from build123d import *

# Parameters (mm, degrees)
SKETCH_R        = 2
SKETCH_W        = 22
SKETCH_H        = 48
PAD_DEPTH       = 7
SKETCH001_W     = 29.4
SKETCH001_H     = 53.5
POCKET_DEPTH    = 6
SKETCH002_R     = 3.5
POCKET001_DEPTH = 3


with BuildPart() as part:
    # Sketch → Pad (new body)
    with BuildSketch(Plane.XY):
        with BuildLine():
            Line((3.870596, 38.332537), (15.423539, 30.665756))
            ThreePointArc((19, 24), (18.049408, 27.782307), (15.423539, 30.665756))
            Line((19, 24), (19, -24))
            ThreePointArc((15.423539, -30.665756), (18.049408, -27.782307), (19, -24))
            Line((15.423539, -30.665756), (3.870596, -38.332537))
            ThreePointArc((-3.870596, -38.332537), (0, -39.5), (3.870596, -38.332537))
            Line((-3.870596, -38.332537), (-15.423539, -30.665756))
            ThreePointArc((-19, -24), (-18.049408, -27.782307), (-15.423539, -30.665756))
            Line((-19, -24), (-19, 24))
            ThreePointArc((-15.423539, 30.665756), (-18.049408, 27.782307), (-19, 24))
            Line((-15.423539, 30.665756), (-3.870596, 38.332537))
            ThreePointArc((3.870596, 38.332537), (0, 39.5), (-3.870596, 38.332537))
        make_face()
        with Locations((0, 32.5)):
            Circle(SKETCH_R, mode=Mode.SUBTRACT)
        with Locations((0, -32.5)):
            Circle(SKETCH_R, mode=Mode.SUBTRACT)
        Rectangle(SKETCH_W, SKETCH_H, mode=Mode.SUBTRACT)
    extrude(amount=PAD_DEPTH)

    # Sketch001 → Pocket (cut)
    with BuildSketch(Plane.XY):
        Rectangle(SKETCH001_W, SKETCH001_H)
    extrude(amount=POCKET_DEPTH, mode=Mode.SUBTRACT)

    # Sketch002 (on Face4 of Pocket) → Pocket001 (cut)
    with BuildSketch(Plane(origin=(0, 0, 0), x_dir=(1, 0, 0), z_dir=(0, 0, -1))):
        with Locations((0, -32.5)):
            Circle(SKETCH002_R)
        with Locations((0, 32.5)):
            Circle(SKETCH002_R)
    extrude(amount=-POCKET001_DEPTH, mode=Mode.SUBTRACT)


solid = part.part
Geometry: final body of the model. Coordinates: model frame, mm. A direction names the side the tool comes from. Give positions to 0.01 mm unless a question says otherwise; leave off trailing zeros. Loops run counter-clockwise (first coordinate to the right, second up) from the corner with the lowest first, then second, coordinate; pieces in that order, holes last. Notation, with made-up numbers: (53, -24) - (76, -24) arc R12 cw to (76, -3) - close; hole circle Ø9 at (81.25, 63). An arc over 180 degrees is marked (long way). One line per question, with ' | ' between items. Start each with the question number.
(1) Ray query, line 1 (X direction, y = 23.5, z = 5); line 2 (Y direction, x = 1.5, z = 5); line 3 (Z direction, x = -12, y = 17). Return the intervals inside material, ascending. Write a range as from..to.
(2) Section query B-B on y = 0.5. Return loops of the section in (x, z).
(3) Reachability of faces 5 (the flat face through (2, 34, 3)), 6 (the flat face through (9.57, 34.55, 3.45)) from +Z, -Z, +X, -X, +Y, -Y: full face, straight path, thin tool, end or side. Return the list, or none.
(4) Section query A-A on x = 0. Return loops of the section in (y, z).
(5) Pull-direction query (Y, two-part tool) for faces 1 (the flat face through (-9.728, 34.445, 3.451)), 2 (the cylindrical face through (0, 29, 1)), 3 (the flat face through (19, 0, 3)), 4 (the cylindrical face through (-0.1, -39.5, 3.5)); classes: released by +Y, released by -Y, zero draft, split by the parting line, or undercut.
(6) Section query C-C on z = 1.25. Return loops of the section in (x, y).
(7) Section query D-D on x = -5. Return loops of the section in (y, z).
(8) Contact query for flat-ended pins moving along their axis: pin 1 (0.8 mm diameter, centred on x = -1, z = 6.5, fed in from +Y); pin 2 (4 mm diameter, centred on x = -4.5, z = 6, fed in from +Y); pin 3 (4 mm diameter, centred on y = -28, z = 3, fed in from -X). Output: stop coordinate, or through.
The answers:
1) line 1: -19..-14.7, 14.7..19 | line 2: -39.34..-33.82, -31.18..-26.75, 26.75..31.18, 33.82..39.34 | line 3: 6..7
2) outline: (-19, 0) - (-14.7, 0) - (-14.7, 6) - (-11, 6) - (-11, 7) - (-19, 7) - close; (11, 6) - (14.7, 6) - (14.7, 0) - (19, 0) - (19, 7) - (11, 7) - close
3) face 5: -Z | face 6: +Z, -Z, +X, +Y
4) outline: (-39.5, 0) - (-36, 0) - (-36, 3) - (-34.5, 3) - (-34.5, 7) - (-39.5, 7) - close; (-30.5, 3) - (-29, 3) - (-29, 0) - (-26.75, 0) - (-26.75, 6) - (-24, 6) - (-24, 7) - (-30.5, 7) - close; (24, 6) - (26.75, 6) - (26.75, 0) - (29, 0) - (29, 3) - (30.5, 3) - (30.5, 7) - (24, 7) - close; (34.5, 3) - (36, 3) - (36, 0) - (39.5, 0) - (39.5, 7) - (34.5, 7) - close
5) face 1: released by +Y | face 2: undercut | face 3: zero draft | face 4: released by -Y
6) outline: (-19, -24) arc R8 ccw to (-15.42, -30.67) - (-3.87, -38.33) arc R7 ccw to (3.87, -38.33) - (15.42, -30.67) arc R8 ccw to (19, -24) - (19, 24) arc R8 ccw to (15.42, 30.67) - (3.87, 38.33) arc R7 ccw to (-3.87, 38.33) - (-15.42, 30.67) arc R8 ccw to (-19, 24) - close; hole (-14.7, -26.75) - (14.7, -26.75) - (14.7, 26.75) - (-14.7, 26.75) - close; hole circle Ø7 at (0, -32.5); hole circle Ø7 at (0, 32.5)
7) outline: (-37.58, 0) - (-26.75, 0) - (-26.75, 6) - (-24, 6) - (-24, 7) - (-37.58, 7) - close; (24, 6) - (26.75, 6) - (26.75, 0) - (37.58, 0) - (37.58, 7) - (24, 7) - close
8) pin 1: y = 39.47 | pin 2: y = 39.04 | pin 3: x = -18.75
